The model under review builds one solid part; all positions refer to its coordinate system, in mm. Coordinates: 2 decimals unless noted, no trailing zeros. Loops run counter-clockwise (first coordinate to the right, second up) from the corner with the lowest first, then second, coordinate; pieces in that order, holes last. Notation, with made-up numbers: (81, -15) - (119, -15) arc R16 cw to (119, 6) - close; hole circle Ø2 at (-20, 12.5). An arc over 180 degrees is marked (long way). One line per item, written item: value. Start each with the question number.
1. To check wall thickness, follow line 1 (Y direction, x = 19, z = 0); line 2 (X direction, y = -3, z = -8); line 3 (Y direction, x = 19, z = -1.5). State the ranges of each line that lie inside material, in increasing order.
2. We need section D-D, the plane x = 3.5. Give the boundary of the cut face in (y, z), then the cut area to 3 significant figures.
3. We need section C-C, the plane z = 10.75. Give the boundary of the cut face in (x, y).
4. We need section B-B, the plane x = 43. Give the boundary of the cut face in (y, z).
5. We need section A-A, the plane y = 0. Give the boundary of the cut face in (x, z), then the cut area to 3 significant figures.
6. Insertion check: P1, Ø12, axis at y = 2, z = -8.5, coming from the -X side; P2, Ø12, axis at y = 6.5, z = -9, coming from the +X side; P3, Ø1, axis at x = 36.5, z = -5, coming from the -Y side; P4, Ø12, axis at x = 7, y = -9, coming from the -Z side. Each pin has a flat end and moves straight along its axis. Give the tip position at first contact, or say it passes through.
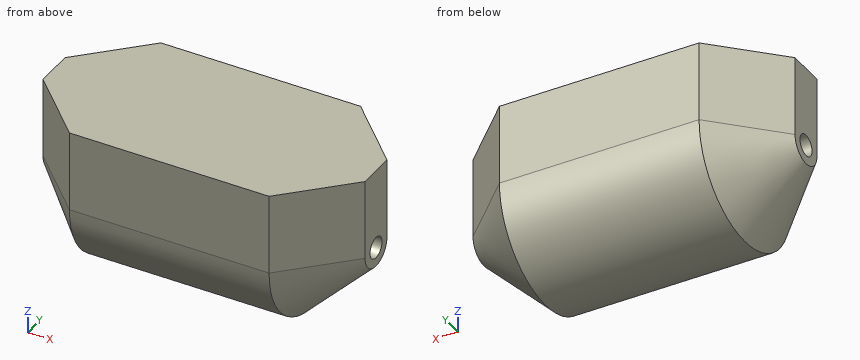
from build123d import *

# Parameters (mm, degrees)
SKETCH1_R           = 1.65
BOSS_EXTRUDE1_DEPTH = 50
CHAMFER1_SIZE       = 9.5


with BuildPart() as part:
    # Sketch1 → Boss-Extrude1 (new body)
    with BuildSketch(Plane(origin=(0, 0, 0), x_dir=(0, 0, -1), z_dir=(1, 0, 0))):
        with BuildLine():
            Line((0, 12.5), (-12.5, 12.5))
            Line((-12.5, 12.5), (-12.5, -12.5))
            Line((-12.5, -12.5), (0, -12.5))
            ThreePointArc((0, -12.5), (12.5, 0), (0, 12.5))
        make_face()
        Circle(SKETCH1_R, mode=Mode.SUBTRACT)
    extrude(amount=BOSS_EXTRUDE1_DEPTH)

    # Chamfer1
    chamfer1_edges = [part.edges().sort_by_distance(p)[0] for p in [
        (50, 12.5, 6.25),
        (50, -12.5, 6.25),
        (0, 12.5, 6.25),
        (0, 0, -12.5),
        (0, -12.5, 6.25),
        (50, 0, -12.5),
    ]]
    chamfer(chamfer1_edges, length=CHAMFER1_SIZE)


solid = part.part
Findings below:
1. line 1: -12.5 to -1.65, 1.65 to 12.5
1. line 2: 5.54 to 44.46
1. line 3: -12.41 to -0.69, 0.69 to 12.41
2. outline: (-6.5, 0) arc R6.5 ccw to (6.5, 0) - (6.5, 12.5) - (-6.5, 12.5) - close; hole circle Ø3.3 at (0, 0)
2. area: 220 mm2
3. outline: (0, -3) - (9.5, -12.5) - (40.5, -12.5) - (50, -3) - (50, 3) - (40.5, 12.5) - (9.5, 12.5) - (0, 3) - close
4. outline: (-10, 0) arc R10 ccw to (10, 0) - (10, 12.5) - (-10, 12.5) - close; hole circle Ø3.3 at (0, 0)
5. outline: (0, -3) - (9.5, -12.5) - (40.5, -12.5) - (50, -3) - (50, -1.65) - (0, -1.65) - close; (0, 1.65) - (50, 1.65) - (50, 12.5) - (0, 12.5) - close
5. area: 995 mm2
6. P1: x = 0
6. P2: x = 47.9
6. P3: y = -11.66
6. P4: z = -11.99
